Verification items for the finished model (mm, model axes). A direction names the side the tool comes from. Give positions to 0.01 mm unless a question says otherwise; leave off trailing zeros. Loops run counter-clockwise (first coordinate to the right, second up) from the corner with the lowest first, then second, coordinate; pieces in that order, holes last. Notation, with made-up numbers: M -34,75.5 L 17,75.5 A20 ccw 17,101.5 Z; hole C 81,19 d6. An arc over 180 degrees is marked long. Use CSV: the item, a comma, the result in double quotes.
from build123d import *

# Parameters (mm, degrees)
F1_DEPTH = 1


with BuildPart() as f1:
    # F0 (on Top) → F1 (new body)
    with BuildSketch(Plane.XY):
        with BuildLine():
            ThreePointArc((0, -2), (-1, -1), (0, 0))
            Line((0, 0), (8, 0))
            Line((8, 0), (8, 2))
            Line((8, 2), (-2, 2))
            Line((-2, 2), (-3.5, 3.2))
            Line((-3.5, 3.2), (-10.5, 3.2))
            Line((-10.5, 3.2), (-12, 2))
            Line((-12, 2), (-22, 2))
            Line((-22, 2), (-22, 0))
            Line((-22, 0), (-14, 0))
            ThreePointArc((-14, 0), (-13, -1), (-14, -2))
            Line((-14, -2), (-22, -2))
            Line((-22, -2), (-22, -4))
            Line((-22, -4), (-12.707107, -4))
            ThreePointArc((-12.707107, -4), (-12.207107, -4.207107), (-12, -4.707107))
            Line((-12, -4.707107), (-12, -5))
            Line((-12, -5), (-2, -5))
            Line((-2, -5), (-2, -4.707107))
            ThreePointArc((-2, -4.707107), (-1.792893, -4.207107), (-1.292893, -4))
            Line((-1.292893, -4), (8, -4))
            Line((8, -4), (8, -2))
            Line((8, -2), (0, -2))
        make_face()
        with BuildLine():
            Line((-4.6, -3.4), (-9.4, -3.4))
            ThreePointArc((-9.4, -3.4), (-10.107107, -3.107107), (-10.4, -2.4))
            Line((-10.4, -2.4), (-10.4, 0.6))
            ThreePointArc((-10.4, 0.6), (-10.107107, 1.307107), (-9.4, 1.6))
            Line((-9.4, 1.6), (-4.6, 1.6))
            ThreePointArc((-4.6, 1.6), (-3.892893, 1.307107), (-3.6, 0.6))
            Line((-3.6, 0.6), (-3.6, -2.4))
            ThreePointArc((-3.6, -2.4), (-3.892893, -3.107107), (-4.6, -3.4))
        make_face(mode=Mode.SUBTRACT)
    extrude(amount=F1_DEPTH)


solid = f1.part
(1) Tool access check on faces 1 (the flat face through (-16.9, 2, 0.5)), 2 (the cylindrical face through (-3.885, -3.099, 0.493)), 3 (the flat face through (-17.9, -2, 0.5)), 4 (the flat face through (-17.4, -4, 0.5)). Record the directions out of +Z, -Z, +X, -X, +Y, -Y that give a thin tool (end or side, any length) a straight path to the whole face; none if there is none.
Calculated:
face 1,"+Z, -Z, -X, +Y"
face 2,"+Z, -Z"
face 3,"+Z, -Z, -X"
face 4,"+Z, -Z, -X, -Y"
(2) Section check C-C on y = -0.25. Record the cut outline in (x, z).
Calculated:
outline,"M -13.34,0 L -10.4,0 L -10.4,1 L -13.34,1 Z; M -3.6,0 L -0.66,0 L -0.66,1 L -3.6,1 Z"
(3) Depth check by flat-ended pin: pin 1 Ø0.5 at (x, z) = (-19, 0.5) entering from -Y; pin 2 Ø0.5 at (x, z) = (-19, 0.5) entering from +Y. Enter the tip coordinate at first touch or a pass-through.
Calculated:
pin 1,"stops at y = -4"
pin 2,"stops at y = 2"
(4) Section check D-D on y = 2.75. Record the cut outline in (x, z), plus the area to 4 significant figures.
Calculated:
outline,"M -11.06,0 L -2.94,0 L -2.94,1 L -11.06,1 Z"
area,"8.125 mm²"
(5) Mould release check, pull along X, two halves, no side actions. Record for faces 5 (the flat face through (-18.1, 0, 0.5)), 6 (the flat face through (-22, 1, 0.5)), 7 (the flat face through (-7, -3.4, 0.5)), 8 (the flat face through (-10.4, -0.9, 0.5)): released by +X, released by -X, zero draft, split by the parting line, or undercut.
Calculated:
face 5,"zero draft"
face 6,"released by -X"
face 7,"undercut"
face 8,"undercut"
(6) Scan lines: L1, parallel to Y at x = -19, z = 0.5; L2, parallel to Y at x = -6.75, z = 0.6; L3, parallel to X at y = -2.25, z = 0.25. Record each from-to range of solid material in increasing order. Write a range as from..to.
Calculated:
L1,"y = -4..-2, 0..2"
L2,"y = -5..-3.4, 1.6..3.2"
L3,"x = -22..-10.4, -3.6..8"
(7) Section check A-A on x = -18.75. Record the cut outline in (y, z).
Calculated:
outline,"M -4,0 L -2,0 L -2,1 L -4,1 Z; M 0,0 L 2,0 L 2,1 L 0,1 Z"
